```python
from build123d import *

# Parameters (mm, degrees)
F1_DEPTH = 6.35
F2_R     = 2
F3_R     = 4


with BuildPart() as f1:
    # F0 (on Top) → F1 (new body)
    with BuildSketch(Plane.XY):
        with BuildLine():
            Line((-26, 0), (0, 0))
            Line((0, 0), (-1.4851485149, 10))
            Line((-1.4851485149, 10), (-13.2425078277, 10))
            ThreePointArc((-13.2425078277, 10), (-15.3638281713, 9.1213203436), (-17.4851485149, 10))
            ThreePointArc((-17.4851485149, 10), (-18.3638281713, 12.1213203436), (-17.4851485149, 14.2426406871))
            Line((-17.4851485149, 14.2426406871), (-17.4851485149, 25.9573593129))
            ThreePointArc((-17.4851485149, 25.9573593129), (-18.3638281713, 28.0786796564), (-17.4851485149, 30.2))
            ThreePointArc((-17.4851485149, 30.2), (-15.3638281713, 31.0786796564), (-13.2425078277, 30.2))
            Line((-13.2425078277, 30.2), (-4.4851485149, 30.2))
            Line((-4.4851485149, 30.2), (-11.2425742574, 75.7))
            Line((-11.2425742574, 75.7), (-36.7524752475, 75.7))
            Line((-36.7524752475, 75.7), (-35.2673267327, 65.7))
            Line((-35.2673267327, 65.7), (-23.5099674198, 65.7))
            ThreePointArc((-23.5099674198, 65.7), (-21.3886470762, 66.5786796564), (-19.2673267327, 65.7))
            ThreePointArc((-19.2673267327, 65.7), (-18.6170084787, 64.7267299535), (-18.3886470762, 63.5786796564))
            ThreePointArc((-18.3886470762, 63.5786796564), (-18.6170084787, 62.4306293593), (-19.2673267327, 61.4573593129))
            Line((-19.2673267327, 61.4573593129), (-19.2673267327, 46.4426406871))
            ThreePointArc((-19.2673267327, 46.4426406871), (-18.6170084787, 45.4693706407), (-18.3886470762, 44.3213203436))
            ThreePointArc((-18.3886470762, 44.3213203436), (-18.6170084787, 43.1732700465), (-19.2673267327, 42.2))
            ThreePointArc((-19.2673267327, 42.2), (-21.3886470762, 41.3213203436), (-23.5099674198, 42.2))
            Line((-23.5099674198, 42.2), (-32.2673267327, 42.2))
            Line((-32.2673267327, 42.2), (-26, 0))
        make_face()
    extrude(amount=F1_DEPTH)

    # F2
    f2_edges = [f1.edges().sort_by_distance(p)[0] for p in [
        (-4.485149, 30.2, 3.175),
        (-36.752475, 75.7, 3.175),
        (-35.267327, 65.7, 3.175),
        (-32.267327, 42.2, 3.175),
        (-11.242574, 75.7, 3.175),
        (-1.485149, 10, 3.175),
        (0, 0, 3.175),
        (-26, 0, 3.175),
    ]]
    fillet(f2_edges, radius=F2_R)

    # F3
    f3_edges = [f1.edges().sort_by_distance(p)[0] for p in [
        (-23.509967, 65.7, 3.175),
        (-19.267327, 61.457359, 3.175),
        (-19.267327, 46.442641, 3.175),
        (-23.509967, 42.2, 3.175),
        (-13.242508, 30.2, 3.175),
        (-17.485149, 25.957359, 3.175),
        (-17.485149, 14.242641, 3.175),
        (-13.242508, 10, 3.175),
    ]]
    fillet(f3_edges, radius=F3_R)


solid = f1.part
```
For this review, take the finished solid that the model builds, in its own axes (mm). A direction names the side the tool comes from. Round coordinates to 2 decimals unless told otherwise and drop trailing zeros. Write each loop counter-clockwise with the first axis right and the second up, starting at its lowest first coordinate (ties: lowest second). Pieces come first, ordered by that corner, then holes. Notation, with made-up numbers: (-1, -21) - (18, -21) arc R13 cw to (18, -14) - close; hole circle Ø5 at (58, 29). An arc over 180 degrees is marked (long way). Write each question's results on one line, items separated by ' | '.
Item 1: Take a section at A-A on x = -10. State the section outline as (y, z) points, then the cut area to 3 significant figures.
Calculated:
outline: (0, 0) - (10, 0) - (10, 6.35) - (0, 6.35) - close; (30.2, 0) - (67.33, 0) - (67.33, 6.35) - (30.2, 6.35) - close | area: 299 mm^2
Item 2: Take a section at D-D on y = 71. State the section outline as (x, z) points, then the cut area to 3 significant figures.
Calculated:
outline: (-36.05, 0) - (-10.54, 0) - (-10.54, 6.35) - (-36.05, 6.35) - close | area: 162 mm^2
Item 3: Draft analysis for pull direction Y (two halves, no side actions). For faces 6 (the face through (-31.45, 41.52, 3.22)), 7 (the face through (-19, 38, 0)), 8 (the face through (-11.646, 75.201, 3.219)), state which applies: pulls with the +Y half, pulls with the -Y half, needs draft (parallel to the pull), parting line crosses it, or undercut.
Calculated:
face 6: undercut | face 7: needs draft | face 8: pulls with the +Y half
Item 4: Take a section at B-B on x = -22. State the section outline as (y, z) points, then the cut area to 3 significant figures.
Calculated:
outline: (0, 0) - (41.38, 0) - (41.38, 6.35) - (0, 6.35) - close; (66.52, 0) - (75.7, 0) - (75.7, 6.35) - (66.52, 6.35) - close | area: 321 mm^2
Item 5: Take a section at C-C on y = 29. State the section outline as (x, z) points.
Calculated:
outline: (-30.31, 0) - (-18.22, 0) - (-18.22, 6.35) - (-30.31, 6.35) - close
Item 6: For pin 1 (1.9 mm diameter, centred on x = -27, z = 2.5, fed in from -Y); pin 2 (2 mm diameter, centred on y = 13, z = 2, fed in from +X); pin 3 (3 mm diameter, centred on y = 53.5, z = 2, fed in from -X), all flat-tipped, find the tip position at first contact; note any pin that passes through.
Calculated:
pin 1: stops at y = 1.08 | pin 2: stops at x = -17.78 | pin 3: stops at x = -19.27
Item 7: To check wall thickness, follow line 1 along Y through (x, z) = (-12.5, 2.5); line 2 along Y through (x, z) = (-12, 2.75); line 3 along X through (y, z) = (49, 3.5). State the ranges of each line that lie inside material, in increasing order. Write a range as from..to.
Calculated:
line 1: y = 0..9.96, 30.24..75.64 | line 2: y = 0..10, 30.2..75.45 | line 3: x = -19.27..-7.28
Item 8: For faces 1 (the face through (-25.6, 0.5, 3.2)), 2 (the face through (-17.616, 14.501, 3.219)), 3 (the face through (-12.957, 9.876, 3.219)), 4 (the face through (-19, 38, 6.35)), 5 (the face through (-29, 65.7, 3)), list the 3-axis set-ups (+Z, -Z, +X, -X, +Y, -Y) from which the entire face can be reached by the end or side of a thin tool; tool diameter is ignored.
Calculated:
face 1: +Z, -Z, -X, -Y | face 2: +Z, -Z, +X | face 3: +Z, -Z | face 4: +Z, +X, -X, +Y, -Y | face 5: +Z, -Z, -X
